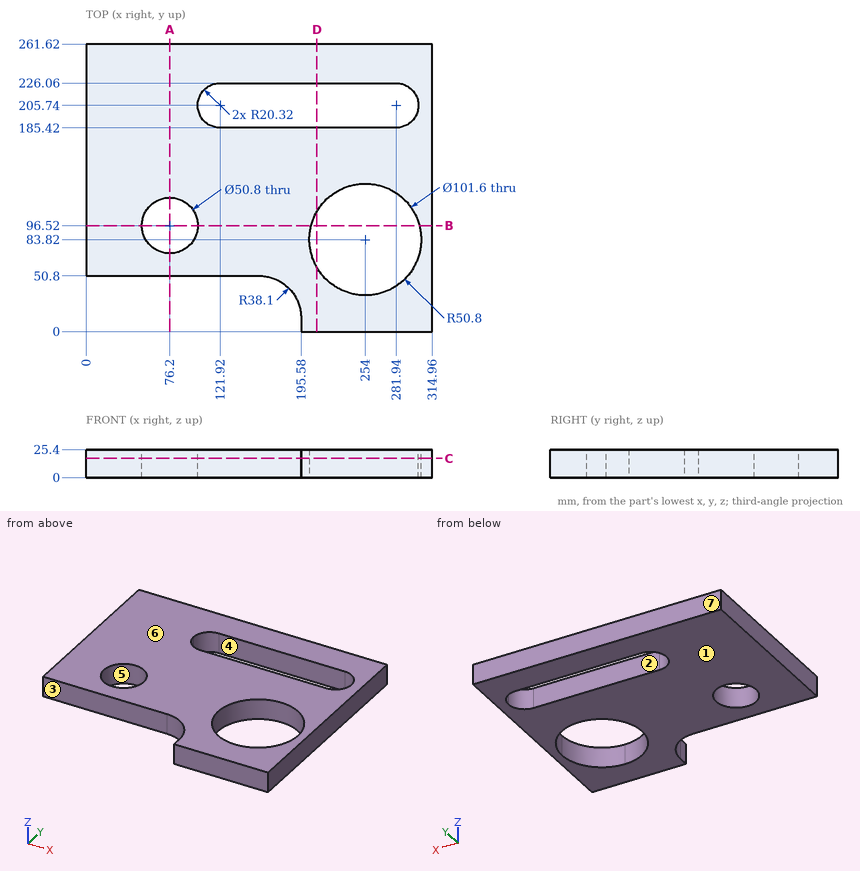
Study the drawing (mm; zero at the part's minimum x, y, z) and answer. A direction names the side the tool comes from. Give positions to 0.01 mm unless a question says otherwise; leave off trailing zeros. Write each loop counter-clockwise with the first axis right and the second up, starting at its lowest first coordinate (ties: lowest second). Pieces come first, ordered by that corner, then holes. Notation, with made-up numbers: (-16.75, 86) -> (5.25, 86) arc R19 cw to (5.25, 107) -> close; hole circle Ø3 at (56, -18.75). An arc over 180 degrees is marked (long way). Write item = value, one per line. Start each with the question number.
1) The part is cut by section B-B, the plane y = 96.52. Determine the outline of the cut face in (x, z), and give its area (3 significant figures).
2) Each of these flat-tipped pins is pushed along its axis until it touches: pin 1 (1 mm diameter, centred on x = 105, z = 17, fed in from -Y); pin 2 (6.5 mm diameter, centred on y = 8, z = 6.5, fed in from -X). Where does it stop, or does it pass through?
3) Straight lines are drawn through the part: line 1 along Y through (x, z) = (254, 5.5); line 2 along X through (y, z) = (83.82, 6.75); line 3 along X through (y, z) = (88.5, 3.25). For each, find the intervals that lie inside material, in ascending order.
4) The part is cut by section D-D, the plane x = 210. Determine the outline of the cut face in (y, z), and give its area (3 significant figures).
5) The part is cut by section A-A, the plane x = 76.2. Determine the outline of the cut face in (y, z), and give its area (3 significant figures).
6) The part is cut by section C-C, the plane z = 17.5. Determine the outline of the cut face in (x, y), and give its area (3 significant figures).
7) Determine the mould class of the marked faces 4, 5, 6 and 7 for opening direction Y: +Y half, -Y half, draft (parallel to the pull), parting line (faces both ways), or undercut.
8) Which of the six approach directions +Z, -Z, +X, -X, +Y, -Y give full straight-line access (tool end or side, diameter ignored) to the marked faces 1, 2 and 3?
Solutions:
q1.outline = (0, 0) -> (50.8, 0) -> (50.8, 25.4) -> (0, 25.4) -> close; (101.6, 0) -> (204.81, 0) -> (204.81, 25.4) -> (101.6, 25.4) -> close; (303.19, 0) -> (314.96, 0) -> (314.96, 25.4) -> (303.19, 25.4) -> close
q1.area = 4,210 mm²
q2.pin_1 = 50.8
q2.pin_2 = 195.58
q3.line_1 = 0 to 33.02, 134.62 to 185.42, 226.06 to 261.62
q3.line_2 = 0 to 54.2, 98.2 to 203.2, 304.8 to 314.96
q3.line_3 = 0 to 52.1, 100.3 to 203.42, 304.58 to 314.96
q4.outline = (0, 0) -> (58.43, 0) -> (58.43, 25.4) -> (0, 25.4) -> close; (109.21, 0) -> (185.42, 0) -> (185.42, 25.4) -> (109.21, 25.4) -> close; (226.06, 0) -> (261.62, 0) -> (261.62, 25.4) -> (226.06, 25.4) -> close
q4.area = 4,320 mm²
q5.outline = (50.8, 0) -> (71.12, 0) -> (71.12, 25.4) -> (50.8, 25.4) -> close; (121.92, 0) -> (261.62, 0) -> (261.62, 25.4) -> (121.92, 25.4) -> close
q5.area = 4,060 mm²
q6.outline = (0, 50.8) -> (157.48, 50.8) arc R38.1 cw to (195.58, 12.7) -> (195.58, 0) -> (314.96, 0) -> (314.96, 261.62) -> (0, 261.62) -> close; hole circle Ø50.8 at (76.2, 96.52); hole (101.6, 205.74) arc R20.32 ccw to (121.92, 185.42) -> (281.94, 185.42) arc R20.32 ccw to (302.26, 205.74) arc R20.32 ccw to (281.94, 226.06) -> (121.92, 226.06) arc R20.32 ccw to start; hole (254, 33.02) arc R50.8 ccw to (304.8, 83.82) arc R50.8 ccw (long way) to start
q6.area = 54,800 mm²
q7.face_4 = undercut
q7.face_5 = undercut
q7.face_6 = draft
q7.face_7 = +Y half
q8.face_1 = -Z, +X, -X, +Y, -Y
q8.face_2 = +Z, -Z
q8.face_3 = +Z, -Z, -X, -Y
